from build123d import *

# Parameters (mm, degrees)
BOSS_EXTRUDE1_DEPTH = 6
SKETCH3_W           = 1.3
SKETCH3_H           = 16.5
BOSS_EXTRUDE2_DEPTH = 2.2
SKETCH4_W           = 1.3
SKETCH4_H           = 16.5
BOSS_EXTRUDE3_DEPTH = 2.2
BOSS_EXTRUDE4_DEPTH = 24
FILLET1_R           = 3
SKETCH6_R           = 2.1
CUT_EXTRUDE1_DEPTH  = 24
SKETCH7_R           = 2.1
CUT_EXTRUDE2_DEPTH  = 24


with BuildPart() as part:
    # Sketch1 → Boss-Extrude1 (new body)
    with BuildSketch(Plane(origin=(0, 0, 0), x_dir=(1, 0, 0), z_dir=(0, 1, 0))):
        Polygon((0, 0), (0, 26), (5, 26), (5, 5), (26, 5), (26, 0), align=None)
    extrude(amount=BOSS_EXTRUDE1_DEPTH)

    # Sketch3 → Boss-Extrude2 (add)
    with BuildSketch(Plane(origin=(0, 6, 0), x_dir=(1, 0, 0), z_dir=(0, 1, 0))):
        with Locations((2.15, 17.75)):
            Rectangle(SKETCH3_W, SKETCH3_H)
    extrude(amount=BOSS_EXTRUDE2_DEPTH)

    # Sketch4 → Boss-Extrude3 (add)
    with BuildSketch(Plane.XZ):
        with Locations((2.15, -17.75)):
            Rectangle(SKETCH4_W, SKETCH4_H)
    extrude(amount=BOSS_EXTRUDE3_DEPTH)

    # Sketch5 → Boss-Extrude4 (add)
    with BuildSketch(Plane(origin=(26, 0, 0), x_dir=(0, 0, -1), z_dir=(1, 0, 0))):
        Polygon((3.75, 6), (3.75, 8), (0, 6), align=None)
        Polygon((3.75, 0), (3.75, -2), (0, 0), align=None)
    extrude(amount=-BOSS_EXTRUDE4_DEPTH)

    # Fillet1
    fillet1_edges = [part.edges().sort_by_distance(p)[0] for p in [
        (5, 3, -5),
    ]]
    fillet(fillet1_edges, radius=FILLET1_R)

    # Sketch6 → Cut-Extrude1 (cut)
    with BuildSketch(Plane(origin=(0, 0, -5), x_dir=(-1, 0, 0), z_dir=(0, 0, -1))):
        with Locations((-22.079, 3)):
            Circle(SKETCH6_R)
    extrude(amount=-CUT_EXTRUDE1_DEPTH, mode=Mode.SUBTRACT)

    # Sketch7 → Cut-Extrude2 (cut)
    with BuildSketch(Plane(origin=(5, 0, 0), x_dir=(0, 0, -1), z_dir=(1, 0, 0))):
        with Locations((22.079, 3)):
            Circle(SKETCH7_R)
    extrude(amount=-CUT_EXTRUDE2_DEPTH, mode=Mode.SUBTRACT)


solid = part.part
Geometry check sheet. Reference: the model listing, model coordinates, mm. A direction names the side the tool comes from. Give positions to 0.01 mm unless a question says otherwise; leave off trailing zeros. Order: outer loops, then holes, each group sorted by start corner. A loop starts at its lowest first (then second) coordinate and runs counter-clockwise, first axis right, second up. Notation, with made-up numbers: M 56.5,86.5 L 101.5,86.5 A19 ccw 101.5,109.5 Z; hole C 80,-30.75 d2. An arc over 180 degrees is marked long. Use a Markdown table: item, result.
Item 1: Material ranges on line 1 along Y through (x, z) = (3.5, -19.25); line 2 along X through (y, z) = (5, -14); line 3 along Z through (x, y) = (15.75, 2.5), recorded low to high.
Answers follow:
| item | result |
|---|---|
| line 1 | y = 0 to 6 |
| line 2 | x = 0 to 5 |
| line 3 | z = -5 to 0 |
Item 2: Section check D-D (y = -1). Record the cut outline in (x, z) (3 decimals).
Answers follow:
| item | result |
|---|---|
| outline | M 1.5,-26 L 2.8,-26 L 2.8,-9.5 L 1.5,-9.5 Z; M 2,-3.75 L 26,-3.75 L 26,-1.875 L 2,-1.875 Z |
Item 3: Section check C-C (z = -10). Record the cut outline in (x, y).
Answers follow:
| item | result |
|---|---|
| outline | M 0,0 L 1.5,0 L 1.5,-2.2 L 2.8,-2.2 L 2.8,0 L 5,0 L 5,6 L 2.8,6 L 2.8,8.2 L 1.5,8.2 L 1.5,6 L 0,6 Z |
Item 4: Section check A-A (y = 3). Record the cut outline in (x, z).
Answers follow:
| item | result |
|---|---|
| outline | M 0,-26 L 5,-26 L 5,-24.18 L 0,-24.18 Z; M 0,-19.98 L 5,-19.98 L 5,-8 A3 cw 8,-5 L 19.98,-5 L 19.98,0 L 0,0 Z; M 24.18,-5 L 26,-5 L 26,0 L 24.18,0 Z |
Item 5: Tool access check on faces 4 (the flat face through (2, -0.8, -2.3)), 5 (the flat face through (1.5, 7, -18)), 6 (the flat face through (2.8, -1, -18)), 7 (the flat face through (5, 3, -17)), 8 (the flat face through (2, 7, -3)). Record the directions out of +Z, -Z, +X, -X, +Y, -Y that give a thin tool (end or side, any length) a straight path to the whole face; none if there is none.
Answers follow:
| item | result |
|---|---|
| face 4 | +Z, -X, -Y |
| face 5 | +Z, -Z, -X, +Y |
| face 6 | -Z, +X, -Y |
| face 7 | -Z, +X, +Y, -Y |
| face 8 | +Z, -X, +Y |
Item 6: Draft check along Z on faces 1 (the flat face through (2, -1, -9.5)), 2 (the flat face through (14.168, -1.014, -1.901)), 3 (the flat face through (2, -2.2, -18)). Enter one of: +Z half, -Z half, draft (parallel to the pull), parting line (faces both ways), or undercut.
Answers follow:
| item | result |
|---|---|
| face 1 | undercut |
| face 2 | +Z half |
| face 3 | draft |
Item 7: Section check B-B (x = 11.75). Record the cut outline in (y, z).
Answers follow:
| item | result |
|---|---|
| outline | M -2,-3.75 L 0,-3.75 L 0,-5 L 6,-5 L 6,-3.75 L 8,-3.75 L 6,0 L 0,0 Z |
Item 8: Depth check by flat-ended pin: P1, Ø0.7, axis at y = 6.5, z = -14.5, coming from the -X side; P2, Ø6, axis at x = 17, y = 1, coming from the -Z side; P3, Ø0.6, axis at y = 7, z = -2.5, coming from the -X side; P4, Ø0.6, axis at y = -1.5, z = -2, coming from the -X side. Enter the tip coordinate at first touch or a pass-through.
Answers follow:
| item | result |
|---|---|
| P1 | stops at x = 1.5 |
| P2 | stops at z = -5 |
| P3 | stops at x = 2 |
| P4 | passes through |
